Read the model definition and answer for the solid it produces. Units are mm, in the model's axes. Face numbers are marked on the shaded views. A direction names the side the tool comes from. Coordinates: 2 decimals unless noted, no trailing zeros. Order: outer loops, then holes, each group sorted by start corner. A loop starts at its lowest first (then second) coordinate and runs counter-clockwise, first axis right, second up.
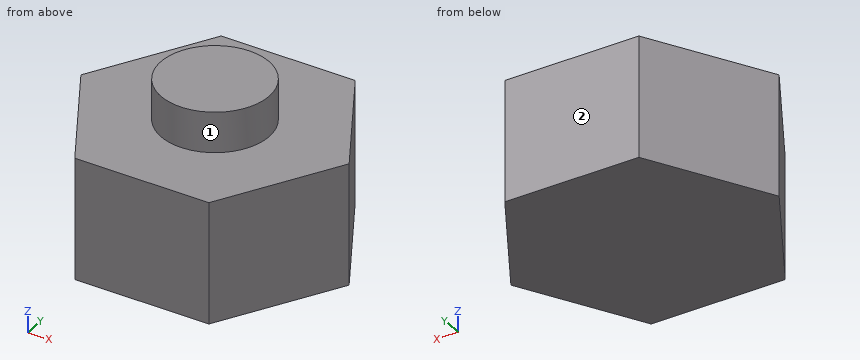
from build123d import *

# Parameters (mm, degrees)
SKETCH_1_R          = 8
EXTRUDE_1_DEPTH     = 24
SKETCH_2_R          = 42
EXTRUDE_2_DEPTH     = 18
SKETCH_3_OUTSIDE_W  = 110.238
SKETCH_3_OUTSIDE_H  = 110.238
CUT_EXTRUDE_1_DEPTH = 63.064482597


with BuildPart() as part:
    # 草图1 → 凸台-拉伸1 (new body)
    with BuildSketch(Plane.XY):
        Circle(SKETCH_1_R)
    extrude(amount=EXTRUDE_1_DEPTH)

    # 草图2 → 凸台-拉伸2 (add)
    with BuildSketch(Plane.XY):
        Circle(SKETCH_2_R)
    extrude(amount=EXTRUDE_2_DEPTH)

    # 草图3 outside → 切除-拉伸1 (cut, through all)
    with BuildSketch(Plane.XY.offset(18)):
        Rectangle(SKETCH_3_OUTSIDE_W, SKETCH_3_OUTSIDE_H)
        Polygon((20, 0), (10, 17.320508076), (-10, 17.320508076), (-20, 0), (-10, -17.320508076), (10, -17.320508076), align=None, mode=Mode.SUBTRACT)
    extrude(amount=-CUT_EXTRUDE_1_DEPTH, mode=Mode.SUBTRACT)


solid = part.part
Q1. Straight lines are drawn through the part: L1, parallel to Z at x = 13.5, y = 1.5; L2, parallel to Y at x = -13, z = 8.25; L3, parallel to X at y = 1.5, z = 4.25. For each, find the intervals that lie inside material, in ascending order.
Q2. The part is cut by section A-A, the plane x = 0. Determine the outline of the cut face in (y, z), then the cut area to 3 significant figures.
Q3. The part is cut by section B-B, the plane z = 11.5. Determine the outline of the cut face in (x, y).
Q4. Which of the six approach directions +Z, -Z, +X, -X, +Y, -Y give full straight-line access (tool end or side, diameter ignored) to the marked faces 1 and 2?
Q5. Each of these flat-tipped pins is pushed along its axis until it touches: P1, Ø3, axis at y = -8, z = 8.5, coming from the -X side; P2, Ø1.5, axis at x = -16, y = 1, coming from the +Z side; P3, Ø4, axis at y = 11.5, z = 8.5, coming from the +X side. Where does it stop, or does it pass through?
Q6. The part is cut by section C-C, the plane y = 2.5. Determine the outline of the cut face in (x, z), then the cut area to 3 significant figures.
Q7. The part is cut by section D-D, the plane y = -12. Determine the outline of the cut face in (x, z), then the cut area to 3 significant figures.
Computed values:
1. L1: z = 0 to 18
1. L2: y = -12.12 to 12.12
1. L3: x = -19.13 to 19.13
2. outline: (-17.32, 0) - (17.32, 0) - (17.32, 18) - (8, 18) - (8, 24) - (-8, 24) - (-8, 18) - (-17.32, 18) - close
2. area: 720 mm2
3. outline: (-20, 0) - (-10, -17.32) - (10, -17.32) - (20, 0) - (10, 17.32) - (-10, 17.32) - close
4. face 1: +Z
4. face 2: +Z, -Z, +X, -X, +Y
5. P1: stops at x = -16.25
5. P2: stops at z = 18
5. P3: stops at x = 14.52
6. outline: (-18.56, 0) - (18.56, 0) - (18.56, 18) - (7.6, 18) - (7.6, 24) - (-7.6, 24) - (-7.6, 18) - (-18.56, 18) - close
6. area: 759 mm2
7. outline: (-13.07, 0) - (13.07, 0) - (13.07, 18) - (-13.07, 18) - close
7. area: 471 mm2
